from build123d import *

# Parameters (mm, degrees)
SKETCH1_R                = 8
SKETCH1_R_2              = 4
BOSS_EXTRUDE1_DEPTH      = 9
BOSS_EXTRUDE1_2_DEPTH    = 9
SKETCH2_R                = 4
BOSS_EXTRUDE3_DEPTH      = 9
FILLET1_R                = 1
CUT_EXTRUDE1_DEPTH       = 214.789616212
SKETCH4_W                = 9
SKETCH4_H                = 27
BOSS_EXTRUDE4_DEPTH      = 75
BOSS_EXTRUDE5_START      = 9
SKETCH5_R                = 25
SKETCH5_R_2              = 4
BOSS_EXTRUDE5_DEPTH      = 9
BOSS_EXTRUDE6_DEPTH      = 4.5
BOSS_EXTRUDE6_DEPTH_BACK = 4.5
BOSS_EXTRUDE7_DEPTH      = 4.5
BOSS_EXTRUDE7_DEPTH_BACK = 4.5
BOSS_EXTRUDE7_START      = -25
SKETCH9_W                = 9
SKETCH9_H                = 7
SKETCH9_H_2              = 9
CUT_EXTRUDE2_DEPTH       = 217.612557346
CUT_EXTRUDE3_DEPTH       = 210.043655728
CUT_EXTRUDE3_DEPTH_BACK  = 210.043655728
SKETCH10_W               = 378.062868676
SKETCH10_H               = 121.353513402
SKETCH10_W_2             = 4.5
SKETCH10_H_2             = 9
SKETCH10_W_3             = 9
SKETCH10_H_3             = 4.5
CUT_EXTRUDE4_DEPTH       = 85.995588121
CUT_EXTRUDE4_DEPTH_BACK  = 85.995588121
SKETCH11_W               = 41.044011783
SKETCH11_H               = 27.30816427
SKETCH11_H_2             = 47.722771097


with BuildPart() as part:
    # Sketch1 → Boss-Extrude1 (new body)
    with BuildSketch(Plane.XY):
        with Locations((-125, 0)):
            Circle(SKETCH1_R)
        with Locations((-125, 0)):
            Circle(SKETCH1_R_2, mode=Mode.SUBTRACT)
    extrude(amount=BOSS_EXTRUDE1_DEPTH)



with BuildPart() as body_2:
    # Sketch1 → Boss-Extrude1 2 (new body)
    with BuildSketch(Plane.XY):
        with Locations((125, 0)):
            Circle(SKETCH1_R)
        with Locations((125, 0)):
            Circle(SKETCH1_R_2, mode=Mode.SUBTRACT)
    extrude(amount=BOSS_EXTRUDE1_2_DEPTH)


with BuildPart() as part_1:
    add(part.part)

    add(body_2.part)  # Boss-Extrude3 merges body 2
    # Sketch2 → Boss-Extrude3 (add)
    with BuildSketch(Plane.XY):
        with BuildLine():
            Line((-175, -75), (125, -75))
            ThreePointArc((125, -75), (130.131670325, -43.377223009), (145.000000492, -14.999999344))
            ThreePointArc((145.000000492, -14.999999344), (143.981414944, 16.269784471), (113.235294528, 22.058823748))
            ThreePointArc((113.235294528, 22.058823748), (25.000000075, 0), (-63.235294395, 22.058823677))
            ThreePointArc((-63.235294395, 22.058823677), (-75.420498385, 24.996463372), (-87.499999896, 21.650635154))
            ThreePointArc((-87.499999896, 21.650635154), (-99.999999954, 18.301270189), (-112.500000024, 21.650635108))
            ThreePointArc((-112.500000024, 21.650635108), (-124.99999995, 25), (-137.49999989, 21.650635158))
            ThreePointArc((-137.49999989, 21.650635158), (-149.999999954, 18.301270189), (-162.50000003, 21.650635112))
            ThreePointArc((-162.50000003, 21.650635112), (-193.705072901, 16.586749162), (-195.000000551, -14.999999265))
            ThreePointArc((-195.000000551, -14.999999265), (-180.13167034, -43.377222962), (-175, -75))
        make_face()
        with Locations((125, 0)):
            Circle(SKETCH2_R, mode=Mode.SUBTRACT)
        with Locations((-175, 0)):
            Circle(SKETCH2_R, mode=Mode.SUBTRACT)
        with Locations((-125, 0)):
            Circle(SKETCH2_R, mode=Mode.SUBTRACT)
        with Locations((-75, 0)):
            Circle(SKETCH2_R, mode=Mode.SUBTRACT)
    extrude(amount=BOSS_EXTRUDE3_DEPTH)

    # Fillet1
    fillet1_edges = [part_1.edges().sort_by_distance(p)[0] for p in [
        (-175, -75, 4.5),
        (125, -75, 4.5),
    ]]
    fillet(fillet1_edges, radius=FILLET1_R)

    # Sketch3 → Cut-Extrude1 (cut, through all)
    with BuildSketch(Plane.XY):
        Polygon((25, 0), (25, -75), (150, -75), (150, 25), (25, 25), align=None)
    extrude(amount=CUT_EXTRUDE1_DEPTH, mode=Mode.SUBTRACT)

    # Sketch4 → Boss-Extrude4 (add)
    with BuildSketch(Plane.XZ.offset(75)):
        with Locations((25, -4.5)):
            Rectangle(SKETCH4_W, SKETCH4_H)
    extrude(amount=-BOSS_EXTRUDE4_DEPTH)

    # Sketch5 → Boss-Extrude5 (add)
    # profile 1 of 4: a face of its own
    with BuildSketch(Plane(origin=(0, 0, -18), x_dir=(-1, 0, 0), z_dir=(0, 0, -1)).offset(BOSS_EXTRUDE5_START)):
        with BuildLine():
            ThreePointArc((-145.000000304, -14.999999594), (-130.131670275, -43.377223158), (-125, -75))
            Line((-125, -75), (-29.5, -75))
            Line((-29.5, -75), (-29.5, 0))
            Line((-29.5, 0), (-100, 0))
            ThreePointArc((-100, 0), (-117.09430609, -23.717082532), (-145.000000304, -14.999999594))
        make_face()
    # profile 2 of 4: a face of its own
    with BuildSketch(Plane(origin=(0, 0, -18), x_dir=(-1, 0, 0), z_dir=(0, 0, -1)).offset(BOSS_EXTRUDE5_START)):
        with Locations((-125, 0)):
            Circle(SKETCH5_R)
        with Locations((-125, 0)):
            Circle(SKETCH5_R_2, mode=Mode.SUBTRACT)
    # profile 3 of 4: a face of its own
    with BuildSketch(Plane(origin=(0, 0, -18), x_dir=(-1, 0, 0), z_dir=(0, 0, -1)).offset(BOSS_EXTRUDE5_START)):
        Polygon((-29.5, 0), (-29.5, -75), (-20.5, -75), (-20.5, 0), (-25, 0), align=None)
    # profile 4 of 4: a face of its own
    with BuildSketch(Plane(origin=(0, 0, -18), x_dir=(-1, 0, 0), z_dir=(0, 0, -1)).offset(BOSS_EXTRUDE5_START)):
        with BuildLine():
            Line((-100, 0), (-29.5, 0))
            Line((-29.5, 0), (-25, 0))
            ThreePointArc((-25, 0), (-70.475429529, 5.598281181), (-113.235293817, 22.058823369))
            ThreePointArc((-113.235293817, 22.058823369), (-103.56267677, 12.86239374), (-100, 0))
        make_face()
    extrude(amount=-BOSS_EXTRUDE5_DEPTH)

    # Sketch7 → Boss-Extrude6 (add, two sides: drawn at the far end of the back side and taken through both)
    with BuildSketch(Plane(origin=(0, -25, 0), x_dir=(1, 0, 0), z_dir=(0, 1, 0)).offset(-BOSS_EXTRUDE6_DEPTH_BACK)):
        with BuildLine():
            Line((56.5, 18), (29.5, 18))
            Line((29.5, 18), (29.5, -9))
            ThreePointArc((29.5, -9), (48.591883092, -1.091883092), (56.5, 18))
        make_face()
        with BuildLine():
            Line((-6.5, 0), (20.5, 0))
            Line((20.5, 0), (20.5, 27))
            ThreePointArc((20.5, 27), (1.408116908, 19.091883092), (-6.5, 0))
        make_face()
    extrude(amount=BOSS_EXTRUDE6_DEPTH + BOSS_EXTRUDE6_DEPTH_BACK)

    # Sketch7<3> → Boss-Extrude7 (add, two sides: drawn at the far end of the back side and taken through both)
    with BuildSketch(Plane(origin=(0, -25, 0), x_dir=(1, 0, 0), z_dir=(0, 1, 0)).offset(BOSS_EXTRUDE7_START - BOSS_EXTRUDE7_DEPTH_BACK)):
        with BuildLine():
            Line((56.5, 18), (29.5, 18))
            Line((29.5, 18), (29.5, -9))
            ThreePointArc((29.5, -9), (48.591883092, -1.091883092), (56.5, 18))
        make_face()
        with BuildLine():
            Line((-6.5, 0), (20.5, 0))
            Line((20.5, 0), (20.5, 27))
            ThreePointArc((20.5, 27), (1.408116908, 19.091883092), (-6.5, 0))
        make_face()
    extrude(amount=BOSS_EXTRUDE7_DEPTH + BOSS_EXTRUDE7_DEPTH_BACK)

    # Sketch9 → Cut-Extrude2 (cut, through all)
    with BuildSketch(Plane.XY.offset(9)):
        with Locations((-160.208548161, -53.5)):
            Rectangle(SKETCH9_W, SKETCH9_H)
        with Locations((-160.208548161, -70.5)):
            Rectangle(SKETCH9_W, SKETCH9_H_2)
        with Locations((-25.351798772, -53.5)):
            Rectangle(SKETCH9_W, SKETCH9_H)
        with Locations((-25.351798772, -70.5)):
            Rectangle(SKETCH9_W, SKETCH9_H_2)
        with Locations((109.504950616, -53.5)):
            Rectangle(SKETCH9_W, SKETCH9_H)
        with Locations((109.504950616, -70.5)):
            Rectangle(SKETCH9_W, SKETCH9_H_2)
    extrude(amount=-CUT_EXTRUDE2_DEPTH, mode=Mode.SUBTRACT)

    # Sketch10 → Cut-Extrude3 (cut, two sides: drawn at the far end of the back side and taken through both)
    # profile 1 of 11: a face of its own
    with BuildSketch(Plane(origin=(0, -20.5, 0), x_dir=(1, 0, 0), z_dir=(0, 1, 0)).offset(-CUT_EXTRUDE3_DEPTH_BACK)):
        with Locations((-22.824558852, 8.698613075)):
            Rectangle(SKETCH10_W, SKETCH10_H)
        with BuildLine():
            ThreePointArc((-6.5, 0), (-4.122805694, 11.077790383), (2.590180724, 20.204909638))
            ThreePointArc((2.590180724, 20.204909638), (30.603376531, 44.977445399), (56.5, 18))
            ThreePointArc((56.5, 18), (54.122805694, 6.922209617), (47.409819276, -2.204909638))
            ThreePointArc((47.409819276, -2.204909638), (23.974453078, -26.775514483), (-4.955844123, -9))
            Line((-4.955844123, -9), (-6.5, -9))
            Line((-6.5, -9), (-6.5, 0))
        make_face(mode=Mode.SUBTRACT)
    # profile 2 of 11: a face of its own
    with BuildSketch(Plane(origin=(0, -20.5, 0), x_dir=(1, 0, 0), z_dir=(0, 1, 0)).offset(-CUT_EXTRUDE3_DEPTH_BACK)):
        with BuildLine():
            ThreePointArc((47.5, 0), (42.545407685, 15.588457268), (29.5, 25.455844123))
            Line((29.5, 25.455844123), (29.5, 18))
            Line((29.5, 18), (29.5, 13.5))
            Line((29.5, 13.5), (29.5, 9))
            Line((29.5, 9), (29.5, 4.5))
            Line((29.5, 4.5), (29.5, 0))
            Line((29.5, 0), (29.5, -9))
            ThreePointArc((29.5, -9), (39.077772178, -7.244133578), (47.409819276, -2.204909638))
            ThreePointArc((47.409819276, -2.204909638), (47.477445399, -1.103376531), (47.5, 0))
        make_face()
    # profile 3 of 11: a face of its own
    with BuildSketch(Plane(origin=(0, -20.5, 0), x_dir=(1, 0, 0), z_dir=(0, 1, 0)).offset(-CUT_EXTRUDE3_DEPTH_BACK)):
        with BuildLine():
            ThreePointArc((2.590180724, 20.204909638), (10.922227822, 25.244133578), (20.5, 27))
            Line((20.5, 27), (29.5, 27))
            Line((29.5, 27), (29.5, 25.455844123))
            ThreePointArc((29.5, 25.455844123), (42.545407685, 15.588457268), (47.5, 0))
            ThreePointArc((47.5, 0), (47.477445399, -1.103376531), (47.409819276, -2.204909638))
            ThreePointArc((47.409819276, -2.204909638), (54.122805694, 6.922209617), (56.5, 18))
            ThreePointArc((56.5, 18), (30.603376531, 44.977445399), (2.590180724, 20.204909638))
        make_face()
    # profile 4 of 11: a face of its own
    with BuildSketch(Plane(origin=(0, -20.5, 0), x_dir=(1, 0, 0), z_dir=(0, 1, 0)).offset(-CUT_EXTRUDE3_DEPTH_BACK)):
        with Locations((4.75, -4.5)):
            Rectangle(SKETCH10_W_2, SKETCH10_H_2)
    # profile 5 of 11: a face of its own
    with BuildSketch(Plane(origin=(0, -20.5, 0), x_dir=(1, 0, 0), z_dir=(0, 1, 0)).offset(-CUT_EXTRUDE3_DEPTH_BACK)):
        with Locations((25, 15.75)):
            Rectangle(SKETCH10_W_3, SKETCH10_H_3)
    # profile 6 of 11: a face of its own
    with BuildSketch(Plane(origin=(0, -20.5, 0), x_dir=(1, 0, 0), z_dir=(0, 1, 0)).offset(-CUT_EXTRUDE3_DEPTH_BACK)):
        with Locations((25, 6.75)):
            Rectangle(SKETCH10_W_3, SKETCH10_H_3)
    # profile 7 of 11: a face of its own
    with BuildSketch(Plane(origin=(0, -20.5, 0), x_dir=(1, 0, 0), z_dir=(0, 1, 0)).offset(-CUT_EXTRUDE3_DEPTH_BACK)):
        with Locations((25, 2.25)):
            Rectangle(SKETCH10_W_3, SKETCH10_H_3)
    # profile 8 of 11: a face of its own
    with BuildSketch(Plane(origin=(0, -20.5, 0), x_dir=(1, 0, 0), z_dir=(0, 1, 0)).offset(-CUT_EXTRUDE3_DEPTH_BACK)):
        with BuildLine():
            Line((20.5, 0), (11.5, 0))
            Line((11.5, 0), (11.5, -2.124611797))
            ThreePointArc((11.5, -2.124611797), (15.739349233, -5.230249471), (20.5, -7.455844123))
            Line((20.5, -7.455844123), (20.5, 0))
        make_face()
    # profile 9 of 11: a face of its own
    with BuildSketch(Plane(origin=(0, -20.5, 0), x_dir=(1, 0, 0), z_dir=(0, 1, 0)).offset(-CUT_EXTRUDE3_DEPTH_BACK)):
        with BuildLine():
            ThreePointArc((20.5, -7.455844123), (15.739349233, -5.230249471), (11.5, -2.124611797))
            Line((11.5, -2.124611797), (11.5, -9))
            Line((11.5, -9), (20.5, -9))
            Line((20.5, -9), (20.5, -7.455844123))
        make_face()
    # profile 10 of 11: a face of its own
    with BuildSketch(Plane(origin=(0, -20.5, 0), x_dir=(1, 0, 0), z_dir=(0, 1, 0)).offset(-CUT_EXTRUDE3_DEPTH_BACK)):
        with BuildLine():
            Line((20.5, -9), (29.5, -9))
            ThreePointArc((29.5, -9), (24.934246574, -8.611161111), (20.5, -7.455844123))
            Line((20.5, -7.455844123), (20.5, -9))
        make_face()
    # profile 11 of 11: a face of its own
    with BuildSketch(Plane(origin=(0, -20.5, 0), x_dir=(1, 0, 0), z_dir=(0, 1, 0)).offset(-CUT_EXTRUDE3_DEPTH_BACK)):
        with BuildLine():
            ThreePointArc((20.5, -7.455844123), (24.934246574, -8.611161111), (29.5, -9))
            Line((29.5, -9), (29.5, 0))
            Line((29.5, 0), (20.5, 0))
            Line((20.5, 0), (20.5, -7.455844123))
        make_face()
    extrude(amount=CUT_EXTRUDE3_DEPTH + CUT_EXTRUDE3_DEPTH_BACK, mode=Mode.SUBTRACT)

    # Sketch11 → Cut-Extrude4 (cut, two sides: drawn at the far end of the back side and taken through both)
    with BuildSketch(Plane.XY.offset(-CUT_EXTRUDE4_DEPTH_BACK)):
        with Locations((11.617711519, -6.845917865)):
            Rectangle(SKETCH11_W, SKETCH11_H)
        with Locations((11.617711519, -53.361385549)):
            Rectangle(SKETCH11_W, SKETCH11_H_2)
    extrude(amount=CUT_EXTRUDE4_DEPTH + CUT_EXTRUDE4_DEPTH_BACK, mode=Mode.SUBTRACT)


solid = part_1.part
Design review of the part built by this model. Coordinates are the model's own, in mm. A direction names the side the tool comes from. Round coordinates to 2 decimals unless told otherwise and drop trailing zeros. Order: outer loops, then holes, each group sorted by start corner. A loop starts at its lowest first (then second) coordinate and runs counter-clockwise, first axis right, second up.
1) Consider section D-D (x = 5.5). State the section outline as (y, z) points, plus the area to 3 significant figures.
The answers:
outline: (-29.5, -22.45) - (-20.5, -22.45) - (-20.5, 0) - (-29.5, 0) - close
area: 202 mm2
2) Consider section C-C (y = -23). State the section outline as (x, z) points, plus the area to 3 significant figures.
The answers:
outline: (-6.5, 0) arc R27 ccw to (20.5, -27) - (29.5, -27) - (29.5, -18) - (20.5, -18) - (20.5, -13.5) - (29.5, -13.5) - (29.5, -9) - (20.5, -9) - (20.5, 0) - (11.5, 0) - (11.5, 9) - (7, 9) - (7, 0) - (2.5, 0) - (2.5, 9) - (-6.5, 9) - close
area: 816 mm2
3) Consider section A-A (z = 1.5). State the section outline as (x, y) points.
The answers:
outline: (-6.5, -29.5) - (2.5, -29.5) - (2.5, -20.5) - (-6.5, -20.5) - close; (7, -29.5) - (11.5, -29.5) - (11.5, -20.5) - (7, -20.5) - close
4) Machinability: for faces 5 (the flat face through (5, -25, 0)), 6 (the flat face through (16, -25, 0)), 7 (the flat face through (29.5, -25, -23)), 8 (the flat face through (25, -25, -18)), which of the approach directions +Z, -Z, +X, -X, +Y, -Y give a long, thin tool a straight path to every point of the face, cutting with its end or side? Answer none if there is none.
The answers:
face 5: +Z, +Y, -Y
face 6: +Z, +X, +Y, -Y
face 7: +Z, -Z, +X, +Y, -Y
face 8: +X, +Y, -Y
5) For L1, parallel to X at y = -29, z = 1.5; L2, parallel to Z at x = 27.5, y = -27; L3, parallel to X at y = -28.25, z = -1.5, list the stretches that pass through material, from the lowest coordinate up.
The answers:
L1: x = -6.5 to 2.5, 7 to 11.5
L2: z = -27 to -18, -13.5 to -9
L3: x = -6.46 to 20.5
6) Clearance check with flat-ended pins moving along their axes: pin 1 Ø2.5 at (y, z) = (-24.5, 4) entering from +X; pin 2 Ø1.3 at (x, y) = (4, -25) entering from +Z; pin 3 Ø2 at (x, y) = (2, -23) entering from -Z. State where each tip first meets the part, or that it passes through.
The answers:
pin 1: stops at x = 11.5
pin 2: stops at z = 0
pin 3: stops at z = -20.56
7) Draft analysis for pull direction X (two halves, no side actions). For faces 1 (the flat face through (29.5, -25, -11)), 2 (the flat face through (25, -25, -13.5)), 3 (the flat face through (7, -25, 5)), 4 (the flat face through (2.5, -25, 5)), state which applies: released by +X, released by -X, zero draft, split by the parting line, or undercut.
The answers:
face 1: released by +X
face 2: zero draft
face 3: undercut
face 4: undercut
8) Consider section B-B (x = 24). State the section outline as (y, z) points.
The answers:
outline: (-29.5, -27) - (-20.5, -27) - (-20.5, -18) - (-29.5, -18) - close; (-29.5, -13.5) - (-20.5, -13.5) - (-20.5, -9) - (-29.5, -9) - close
